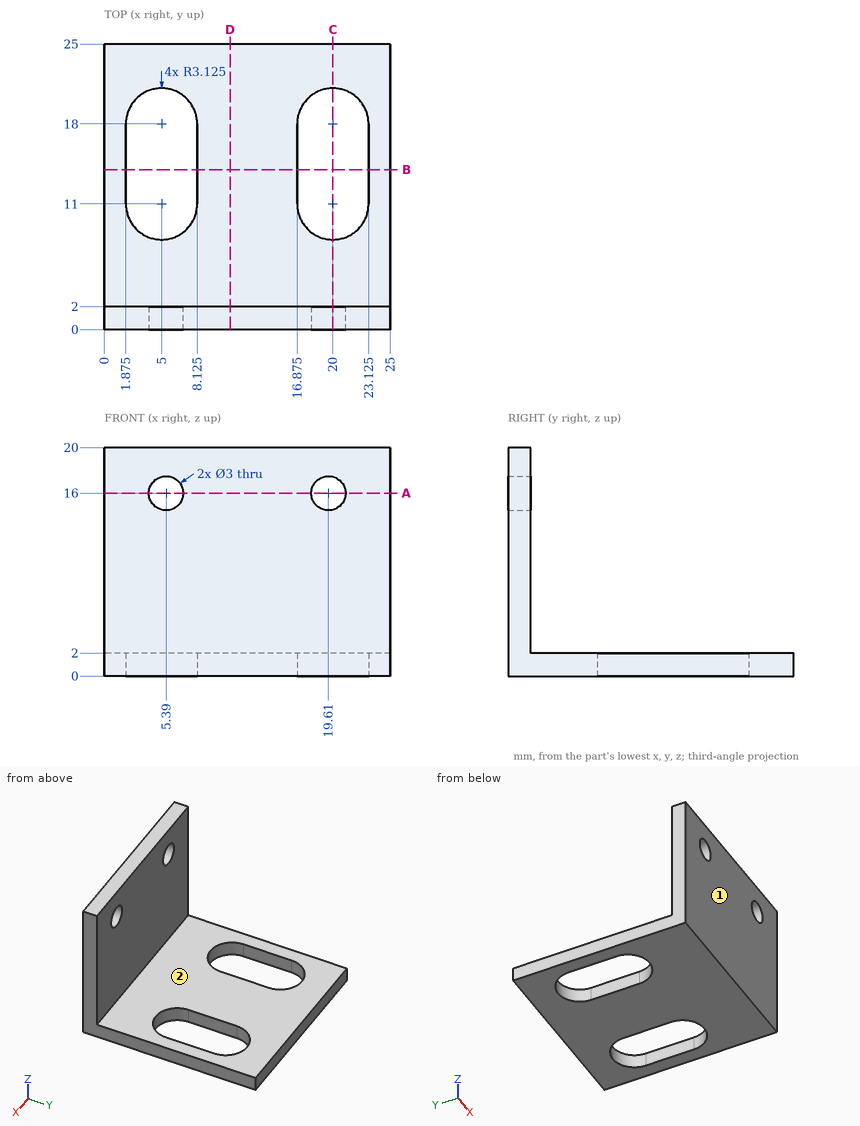
Answer from the drawing. Dimensions are ordinates in mm from the lowest x, y and z of the part. A direction names the side the tool comes from. Give positions to 0.01 mm unless a question says otherwise; leave off trailing zeros. Write each loop counter-clockwise with the first axis right and the second up, starting at its lowest first coordinate (ties: lowest second). Pieces come first, ordered by that corner, then holes.
1) Section D-D (x = 11) is taken. Write down the section's boundary in (y, z).
2) Given P1, Ø1.5, axis at x = 10, y = 9, coming from the +Z side; P2, Ø5, axis at y = 5, z = 13, coming from the -X side, each flat-ended and moving along its own axis, determine where each tip first touches the part or whether it passes through.
3) Section A-A (z = 16) is taken. Write down the section's boundary in (x, y), and give its area (3 significant figures).
4) Find the intervals of material crossed by L1, parallel to Y at x = 13, z = 9; L2, parallel to Z at x = 19.61, y = 1.25, in increasing order.
5) A tool of negligible diameter and unlimited length cuts with its end or side. For the marked faces 1 and 2, from which of +Z, -Z, +X, -X, +Y, -Y can it reach the whole face along a straight path? Write none if from no direction.
6) Section C-C (x = 20) is taken. Write down the section's boundary in (y, z) (3 decimals), and give its area (3 significant figures).
7) Section B-B (y = 14) is taken. Write down the section's boundary in (x, z) (3 decimals).
Response:
1. outline: (0, 0) - (25, 0) - (25, 2) - (2, 2) - (2, 20) - (0, 20) - close
2. P1: stops at z = 2
2. P2: passes through
3. outline: (0, 0) - (3.89, 0) - (3.89, 2) - (0, 2) - close; (6.89, 0) - (18.11, 0) - (18.11, 2) - (6.89, 2) - close; (21.11, 0) - (25, 0) - (25, 2) - (21.11, 2) - close
3. area: 38.0 mm2
4. L1: y = 0 to 2
4. L2: z = 0 to 14.5, 17.5 to 20
5. face 1: +Z, -Z, +X, -X, -Y
5. face 2: +Z, +X, -X, +Y
6. outline: (0, 0) - (7.875, 0) - (7.875, 2) - (2, 2) - (2, 14.552) - (0, 14.552) - close; (0, 17.448) - (2, 17.448) - (2, 20) - (0, 20) - close; (21.125, 0) - (25, 0) - (25, 2) - (21.125, 2) - close
6. area: 53.7 mm2
7. outline: (0, 0) - (1.875, 0) - (1.875, 2) - (0, 2) - close; (8.125, 0) - (16.875, 0) - (16.875, 2) - (8.125, 2) - close; (23.125, 0) - (25, 0) - (25, 2) - (23.125, 2) - close
